Geometry: final body of the model. Coordinates: model frame, mm. A direction names the side the tool comes from. Give positions to 0.01 mm unless a question says otherwise; leave off trailing zeros. Loops run counter-clockwise (first coordinate to the right, second up) from the corner with the lowest first, then second, coordinate; pieces in that order, holes last. Notation, with made-up numbers: (83.25, -7.75) -> (133.25, -7.75) arc R9 ccw to (133.25, 6.25) -> close; hole circle Ø5 at (-19.75, 51.5). An arc over 180 degrees is marked (long way). One line per question, with ' | ' between items. Start each with the question number.
Item 1: Material intervals for line 1 along Z through (x, y) = (6.35, 19.8); line 2 along Z through (x, y) = (10.5, 12.75); line 3 along Y through (x, z) = (6.35, -20.6), sorted ascending. Write a range as [from, to].
Item 2: Set-up query: faces 1 (the flat face through (6, -1.243, 21)), 2 (the flat face through (6, -1.728, -21)), 3 (the flat face through (6, 8, -19.195)). Return all of +Z, -Z, +X, -X, +Y, -Y with unobstructed straight access to the full face (end or side cutting, diameter ignored); none if empty.
Item 3: Mould query, pull axis Y, two halves, no side actions, for faces 4 (the cylindrical face through (3.83, 2.69, -20.67)), 5 (the flat face through (6, 9, -22.192)), 6 (the flat face through (9, 20.804, 0)). Classes: released by +Y, released by -Y, zero draft, split by the parting line, or undercut.
Item 4: Section C-C on z = -0.5. Return loops of the section in (x, y).
Item 5: Pin query (flat end, axial travel): P1, Ø1.5, axis at x = 8.5, z = -2, coming from the -Y side; P2, Ø2.5, axis at x = 8.5, z = 21, coming from the -Y side. Return the tip coordinate at first contact, or that it passes through.
Item 6: Section D-D on y = 5.5. Return loops of the section in (x, z).
Item 7: Section A-A on y = 8.25. Return loops of the section in (x, z), then the cut area to 3 significant figures.
Item 8: Section B-B on x = 6.35. Return loops of the section in (y, z), then the cut area to 3 significant figures.
Autodesk Inventor part; units mm, degrees
ref_plane "YZ Plane" through (0, 0, 0) normal (1, 0, 0) x (0, 1, 0)
ref_plane "XZ Plane" through (0, 0, 0) normal (0, 1, 0) x (-1, 0, 0)
sketch "Sketch1" plane through (0, 0, 0) normal (1, 0, 0) x (0, 1, 0)
  line L0 (-1.2434, 22.2577) -> (20.8038, 22.2577)
  line L1 (20.8038, 22.2577) -> (20.8038, -15.9039)
  line L2 (17.8066, 19.2605) -> (-1.2434, 19.2605)
  line L3 (-1.2434, 19.2605) -> (-1.2434, 22.2577)
  line L4 (20.8038, 22.2577) -> (1.0601, 22.2577)
  line L5 (17.8066, 19.2605) -> (17.8066, -19.1951)
  line L6 (1.0601, -22.1923) -> (20.8038, -22.1923)
  line L7 (20.8038, -22.1923) -> (20.8038, 22.2577)
  line L8 (20.8038, -22.1923) -> (-1.7276, -22.1923)
  line L9 (-1.7276, -22.1923) -> (-1.7276, -19.1951)
  line L10 (-1.7276, -19.1951) -> (17.8066, -19.1951)
  line L11 (20.8038, -19.8757) -> (20.8038, -22.1923)
  point P0 (0, 0)
  dimension "d0" = 2.9972
  dimension "d1" = 19.05
  dimension "d2" = 44.45
  dimension "d3" = 2.9972
extrude "Extrusion1" add sketch "Sketch1" along normal blind 12.7
sketch "Sketch2" plane through (0, -1.2434, 22.2577) normal (0, 0, 1) x (1, 0, 0)
  circle A0 centre (6.35, 5.8657) radius 3.175
  line L0 (0, -0.4843) -> (12.7, -0.4843)
  line L1 (12.7, 22.0472) -> (12.7, 0)
  point P0 (0, 1.2434)
  dimension "d6" = 6.35
  dimension "d7" = 6.35
  dimension "d8" = 6.35
extrude "Extrusion2" cut sketch "Sketch2" against normal through all
sketch "Sketch3" plane through (0, 20.8038, 22.2577) normal (0, 1, 0) x (1, 0, 0)
  line L0 (9.525, 0) -> (3.175, 0)
  line L1 (6.35, 0) -> (6.35, 44.45) construction
  line L2 (0, 44.45) -> (12.7, 44.45)
  circle A0 centre (6.35, 9.525) radius 1.7272
  circle A1 centre (6.35, 22.225) radius 1.7272
  circle A2 centre (6.35, 34.925) radius 1.7272
  point P0 (0, 22.2577)
  dimension "d11" = 3.4544
  dimension "d12" = 12.7
  dimension "d13" = 12.7
hole "Hole1" at (6.35, 20.8038, -12.6673) at (6.35, 20.8038, 0.0327) at (6.35, 20.8038, 12.7327) direction (0, -1, 0) diameter 3.4544 end through all
properties part number "Papa John Bolt Plate" material "Polycarbonate, Clear"
Result sheet:
1) line 1: z = [-22.19, -14.39], [-10.94, -1.69], [1.76, 11.01], [14.46, 22.26] | line 2: z = [-22.19, -19.2], [19.26, 22.26] | line 3: y = [-1.73, 1.45], [7.8, 20.8]
2) face 1: +Z, +X, -X, -Y | face 2: +Z, -Z, +X, -X, -Y | face 3: +X, -X, -Y
3) face 4: undercut | face 5: zero draft | face 6: released by +Y
4) outline: (0, 17.81) -> (4.71, 17.81) -> (4.71, 20.8) -> (0, 20.8) -> close; (7.99, 17.81) -> (12.7, 17.81) -> (12.7, 20.8) -> (7.99, 20.8) -> close
5) P1: stops at y = 17.81 | P2: stops at y = -1.24
6) outline: (0, -22.19) -> (3.3, -22.19) -> (3.3, -19.2) -> (0, -19.2) -> close; (0, 19.26) -> (3.3, 19.26) -> (3.3, 22.26) -> (0, 22.26) -> close; (9.4, -22.19) -> (12.7, -22.19) -> (12.7, -19.2) -> (9.4, -19.2) -> close; (9.4, 19.26) -> (12.7, 19.26) -> (12.7, 22.26) -> (9.4, 22.26) -> close
7) outline: (0, -22.19) -> (12.7, -22.19) -> (12.7, -19.2) -> (0, -19.2) -> close; (0, 19.26) -> (12.7, 19.26) -> (12.7, 22.26) -> (0, 22.26) -> close | area: 76.1 mm²
8) outline: (-1.73, -22.19) -> (1.45, -22.19) -> (1.45, -19.2) -> (-1.73, -19.2) -> close; (-1.24, 19.26) -> (1.45, 19.26) -> (1.45, 22.26) -> (-1.24, 22.26) -> close; (7.8, -22.19) -> (20.8, -22.19) -> (20.8, -14.39) -> (17.81, -14.39) -> (17.81, -19.2) -> (7.8, -19.2) -> close; (7.8, 19.26) -> (17.81, 19.26) -> (17.81, 14.46) -> (20.8, 14.46) -> (20.8, 22.26) -> (7.8, 22.26) -> close; (17.81, -10.94) -> (20.8, -10.94) -> (20.8, -1.69) -> (17.81, -1.69) -> close; (17.81, 1.76) -> (20.8, 1.76) -> (20.8, 11.01) -> (17.81, 11.01) -> close | area: 180 mm²
